from build123d import *

# Parameters (mm, degrees)
F0_R     = 10.95
F0_R_2   = 7.95
F1_DEPTH = 2
F0_R_3   = 6
F2_DEPTH = 2
F0_R_4   = 4.05
F3_DEPTH = 2.5
F0_R_5   = 3.302
F4_DEPTH = 4.75


with BuildPart() as f1:
    # F0 (on Front) → F1 (new body)
    with BuildSketch(Plane.XZ):
        Circle(F0_R)
        Circle(F0_R_2, mode=Mode.SUBTRACT)
    extrude(amount=F1_DEPTH)

    # F0 (on Front) → F2 (join)
    with BuildSketch(Plane.XZ):
        Circle(F0_R_2)
        Circle(F0_R_3, mode=Mode.SUBTRACT)
    extrude(amount=F2_DEPTH)

    # F0 (on Front) → F3 (join)
    with BuildSketch(Plane.XZ):
        Circle(F0_R_3)
        Circle(F0_R_4, mode=Mode.SUBTRACT)
    extrude(amount=F3_DEPTH)

    # F0 (on Front) → F4 (join)
    with BuildSketch(Plane.XZ):
        Circle(F0_R_4)
        Circle(F0_R_5, mode=Mode.SUBTRACT)
    extrude(amount=F4_DEPTH)


solid = f1.part
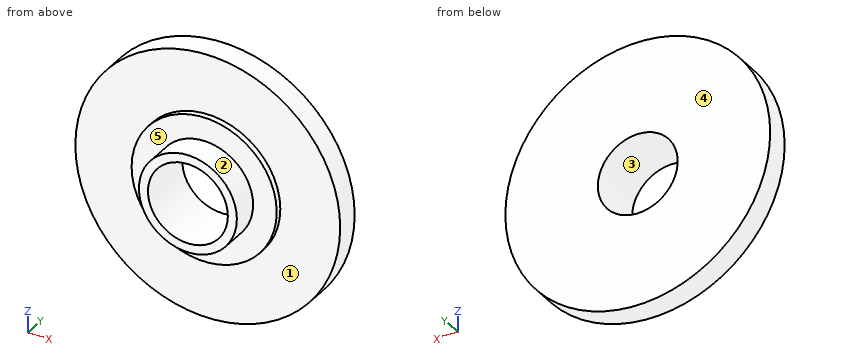
Model file for the job. Use its own axes, mm. Face numbers are marked on the shaded views. A direction names the side the tool comes from. Round coordinates to 2 decimals unless told otherwise and drop trailing zeros. Loops run counter-clockwise (first coordinate to the right, second up) from the corner with the lowest first, then second, coordinate; pieces in that order, holes last. Notation, with made-up numbers: (20.5, -23.5) - (70.5, -23.5) arc R21 cw to (70.5, 4.5) - close; hole circle Ø3 at (77, 0.25). An arc over 180 degrees is marked (long way). Write each question's results on one line, items separated by ' | '.
(1) Saw through at B-B, the plane x = 0. List the corners of the cut face in (y, z), then the cut area to 3 significant figures.
Answer below:
outline: (-4.75, -4.05) - (-2.5, -4.05) - (-2.5, -6) - (-2, -6) - (-2, -10.95) - (0, -10.95) - (0, -3.3) - (-4.75, -3.3) - close; (-4.75, 3.3) - (0, 3.3) - (0, 10.95) - (-2, 10.95) - (-2, 6) - (-2.5, 6) - (-2.5, 4.05) - (-4.75, 4.05) - close | area: 36.7 mm^2
(2) Saw through at D-D, the plane z = 5. List the corners of the cut face in (x, y), then the cut area to 3 significant figures.
Answer below:
outline: (-9.74, -2) - (-3.32, -2) - (-3.32, -2.5) - (3.32, -2.5) - (3.32, -2) - (9.74, -2) - (9.74, 0) - (-9.74, 0) - close | area: 42.3 mm^2
(3) Mould opens along X. For the marked faces 1, 2 and 3 say: released by +X, released by -X, zero draft, split by the parting line, or undercut.
Answer below:
face 1: zero draft | face 2: split by the parting line | face 3: undercut
(4) 3-axis set-ups, long thin cutter, end or side, ignore diameter. For the marked faces 4 and 5: which of +Z, -Z, +X, -X, +Y, -Y reach the whole face in a straight line?
Answer below:
face 4: +Z, -Z, +X, -X, +Y | face 5: -Y
(5) Saw through at A-A, the plane z = 0. List the corners of the cut face in (x, y).
Answer below:
outline: (-10.95, -2) - (-6, -2) - (-6, -2.5) - (-4.05, -2.5) - (-4.05, -4.75) - (-3.3, -4.75) - (-3.3, 0) - (-10.95, 0) - close; (3.3, -4.75) - (4.05, -4.75) - (4.05, -2.5) - (6, -2.5) - (6, -2) - (10.95, -2) - (10.95, 0) - (3.3, 0) - close
(6) Saw through at C-C, the plane y = -0.55. List the corners of the cut face in (x, z), then the cut area to 3 significant figures.
Answer below:
outline: circle Ø21.9 at (0, 0); hole circle Ø6.6 at (0, 0) | area: 342 mm^2
(7) Wall check: L1, parallel to Z at x = 0, y = -2.6; L2, parallel to Z at x = 0, y = -1.2; L3, parallel to Y at x = 3.25, z = -6.25. Give the ranges that are in metal, low to high.
Answer below:
L1: z = -4.05 to -3.3, 3.3 to 4.05 | L2: z = -10.95 to -3.3, 3.3 to 10.95 | L3: y = -2 to 0
(8) Pin check, flat tips, straight feed: pin 1 (2 mm diameter, centred on x = 7.5, z = 8, fed in from -Y); pin 2 (6 mm diameter, centred on x = -8, z = -2.5, fed in from -Y); pin 3 (5.5 mm diameter, centred on x = 0, z = 0, fed in from -Y). Stop position of each tip, or through.
Answer below:
pin 1: stops at y = -2 | pin 2: stops at y = -2.5 | pin 3: passes through
